Build history of the part. All positions in model axes, mm. Face numbers are marked on the shaded views. Round coordinates to 2 decimals unless told otherwise and drop trailing zeros. Order: outer loops, then holes, each group sorted by start corner. A loop starts at its lowest first (then second) coordinate and runs counter-clockwise, first axis right, second up. Notation, with made-up numbers: M -22.75,38 L -16.75,38 A16 ccw -16.75,42 Z; hole C 57,5.25 d6. An arc over 180 degrees is marked long. One line per question, with ' | ' between items. Start each with the question number.
from build123d import *

# Parameters (mm, degrees)
SKETCH_2_R          = 13
EXTRUDE_1_DEPTH     = 4.5
SKETCH_3_R          = 13.5
EXTRUDE_2_DEPTH     = 9.5
SKETCH_4_R          = 12
CUT_EXTRUDE_1_DEPTH = 2
SKETCH_5_R          = 10.172
CUT_EXTRUDE_2_DEPTH = 27
CHAMFER_1_SIZE      = 0.828


with BuildPart() as part:
    # Эскиз2 → Бобышка-Вытянуть1 (new body)
    with BuildSketch(Plane.XY):
        Circle(SKETCH_2_R)
    extrude(amount=EXTRUDE_1_DEPTH)

    # Эскиз3 → Бобышка-Вытянуть2 (add)
    with BuildSketch(Plane.XY.offset(4.5)):
        Circle(SKETCH_3_R)
    extrude(amount=EXTRUDE_2_DEPTH)

    # Эскиз4 → Вырез-Вытянуть1 (cut)
    with BuildSketch(Plane(origin=(0, 0, 0), x_dir=(-1, 0, 0), z_dir=(0, 0, -1))):
        Circle(SKETCH_4_R)
    extrude(amount=-CUT_EXTRUDE_1_DEPTH, mode=Mode.SUBTRACT)

    # Зеркальное отражение4: part across plane


with BuildPart() as part_1:
    add(part.part)
    add(part.part.mirror(Plane.XY.offset(14)))

    # Эскиз5 → Вырез-Вытянуть2 (cut, through all)
    with BuildSketch(Plane(origin=(0, 0, 2), x_dir=(-1, 0, 0), z_dir=(0, 0, -1))):
        Circle(SKETCH_5_R)
    extrude(amount=-CUT_EXTRUDE_2_DEPTH, mode=Mode.SUBTRACT)

    # Фаска1
    chamfer_1_edges = [part_1.edges().sort_by_distance(p)[0] for p in [
        (10.172, 0, 26),
        (10.172, 0, 2),
    ]]
    chamfer(chamfer_1_edges, length=CHAMFER_1_SIZE)


solid = part_1.part
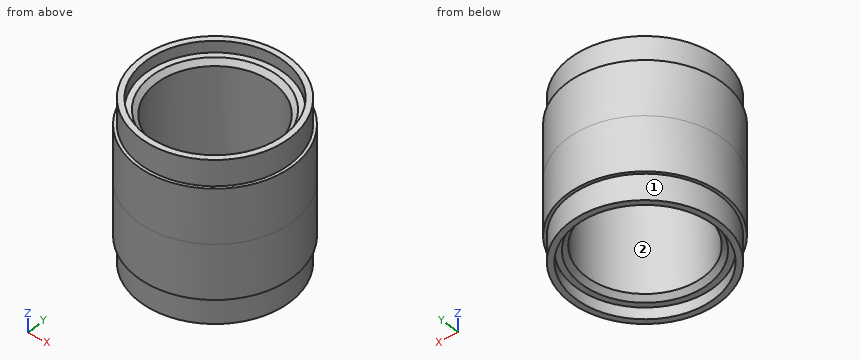
Item 1: Cut at D-D on z = 24. Write the cut outline in (x, y).
Item 2: Cut at C-C on z = 20.25. Write the cut outline in (x, y).
Item 3: Two-plate mould, pull along X, no slides. Class the marked faces 1 and 2: +X half, -X half, draft (parallel to the pull), parting line (faces both ways), or undercut.
Item 4: Wall check: line 1 along Y through (x, z) = (0, 0.45); line 2 along X through (y, z) = (0.25, 24.5); line 3 along Y through (x, z) = (7.5, 20.25). Give the ranges that are in metal, low to high. Write a range as [from, to].
Item 5: Flat gauge pins, fed straight in: pin 1 (12 mm diameter, centred on x = -4.5, y = -3, fed in from -Z); pin 2 (1 mm diameter, centred on x = 6, z = 16, fed in from +Y); pin 3 (2 mm diameter, centred on x = 5, z = 24, fed in from +Y). Where does each tip first touch, or does it go through?
Item 6: Cut at A-A on y = 0. Write the cut outline in (x, z), then the cut area to 3 significant figures.
Results found:
1) outline: C 0,0 d26; hole C 0,0 d20.34
2) outline: C 0,0 d27; hole C 0,0 d20.34
3) face 1: parting line | face 2: undercut
4) line 1: y = [-13, -12], [12, 13] | line 2: x = [-13, -10.17], [10.17, 13] | line 3: y = [-11.22, -6.87], [6.87, 11.22]
5) pin 1: stops at z = 2 | pin 2: stops at y = 12.33 | pin 3: stops at y = 12.85
6) outline: M -13.5,4.5 L -13,4.5 L -13,0 L -12,0 L -12,2 L -11,2 L -10.17,2.83 L -10.17,25.17 L -11,26 L -12,26 L -12,28 L -13,28 L -13,23.5 L -13.5,23.5 Z; M 10.17,2.83 L 11,2 L 12,2 L 12,0 L 13,0 L 13,4.5 L 13.5,4.5 L 13.5,23.5 L 13,23.5 L 13,28 L 12,28 L 12,26 L 11,26 L 10.17,25.17 Z | area: 161 mm^2
